Could you check a few things on this drawing? It's one solid part, dimensions in mm from its lowest x, y, z. A direction names the side the tool comes from. Round coordinates to 2 decimals unless told otherwise and drop trailing zeros. Write each loop counter-clockwise with the first axis right and the second up, starting at its lowest first coordinate (ties: lowest second). Pieces come first, ordered by that corner, then holes. Notation, with made-up numbers: (65, -31.75) -> (75, -31.75) arc R21 ccw to (75, -8.75) -> close; hole circle Ø3 at (4.5, 11.5). An arc over 180 degrees is marked (long way). Answer in a Markdown table with one row per item. Add a question column.
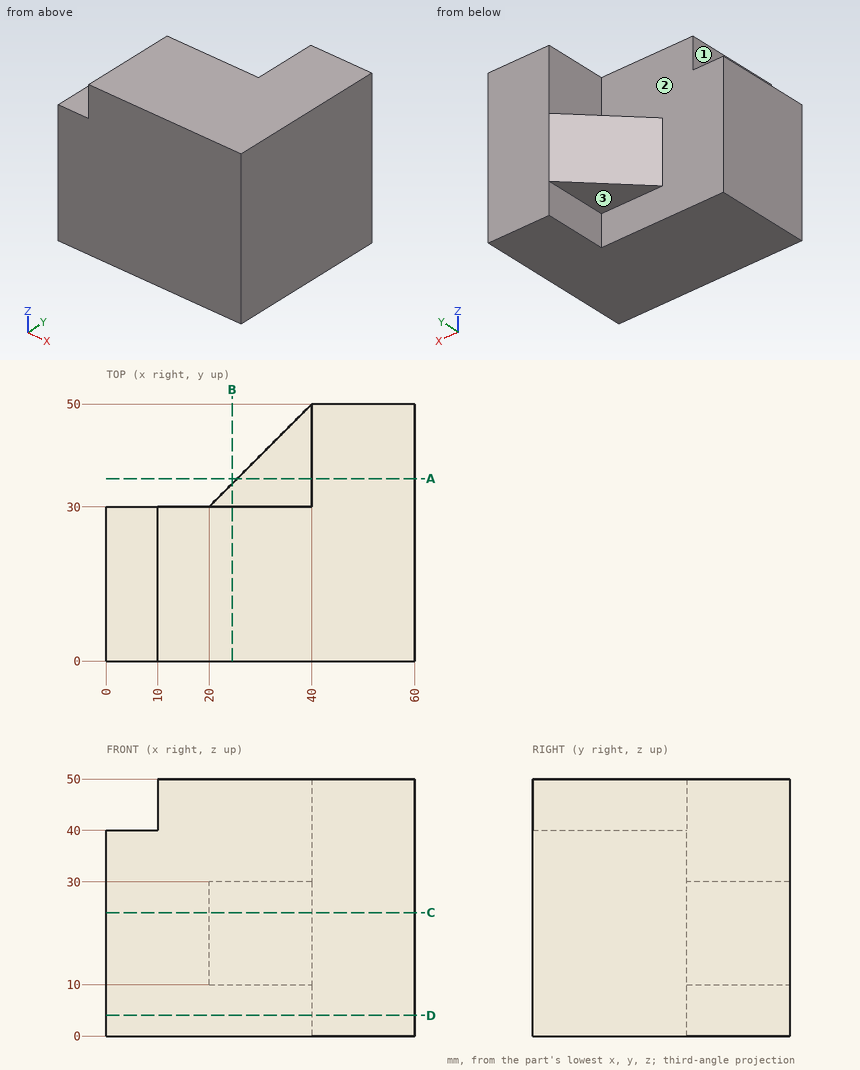
Item 1: If we section it at D-D on z = 4: Please give me the cut outline in (x, y), then the cut area to 3 significant figures.
Item 2: If we section it at A-A on y = 35.5: Please give me the cut outline in (x, z).
Item 3: If we section it at C-C on z = 24: Please give me the cut outline in (x, y), then the cut area to 3 significant figures.
Item 4: For P1, Ø3, axis at x = 43.5, y = 42, coming from the -Z side; P2, Ø16, axis at x = 25.5, y = 44, coming from the +Z side; P3, Ø11, axis at y = 39.5, z = 2.5, coming from the -X side; P4, Ø5, axis at x = 7, z = 24, coming from the +Y side, each with a flat end and sliding along its axis, tell me the tip position at first contact or that it passes through.
Item 5: On a 3-axis mill with a long thin cutter (end or side, diameter ignored), from which of +Z, -Z, +X, -X, +Y, -Y can I reach the whole of each face in a straight line? I mean the marked faces 1, 2 and 3. Say none if no direction works.
Item 6: If we section it at B-B on x = 24.5: Please give me the cut outline in (y, z), then the cut area to 3 significant figures.
Item 7: I need wall thicknesses on line 1 along Y through (x, z) = (7.5, 18); line 2 along X through (y, z) = (23, 40.5); line 3 along X through (y, z) = (39, 34.5). Which ranges of each line are inside material? Lowest first, please. Write a range as from..to.
Results list:
| question | item | result |
|---|---|---|
| 1 | outline | (0, 0) -> (60, 0) -> (60, 50) -> (40, 50) -> (40, 30) -> (0, 30) -> close |
| 1 | area | 2,200 mm² |
| 2 | outline | (25.5, 10) -> (40, 10) -> (40, 0) -> (60, 0) -> (60, 50) -> (40, 50) -> (40, 30) -> (25.5, 30) -> close |
| 3 | outline | (0, 0) -> (60, 0) -> (60, 50) -> (40, 50) -> (20, 30) -> (0, 30) -> close |
| 3 | area | 2,400 mm² |
| 4 | P1 | z = 0 |
| 4 | P2 | z = 30 |
| 4 | P3 | x = 40 |
| 4 | P4 | y = 30 |
| 5 | face 1 | +Z, -X, +Y, -Y |
| 5 | face 2 | -X, +Y |
| 5 | face 3 | -Z, -X, +Y |
| 6 | outline | (0, 0) -> (30, 0) -> (30, 10) -> (34.5, 10) -> (34.5, 30) -> (30, 30) -> (30, 50) -> (0, 50) -> close |
| 6 | area | 1,590 mm² |
| 7 | line 1 | 0..30 |
| 7 | line 2 | 10..60 |
| 7 | line 3 | 40..60 |
